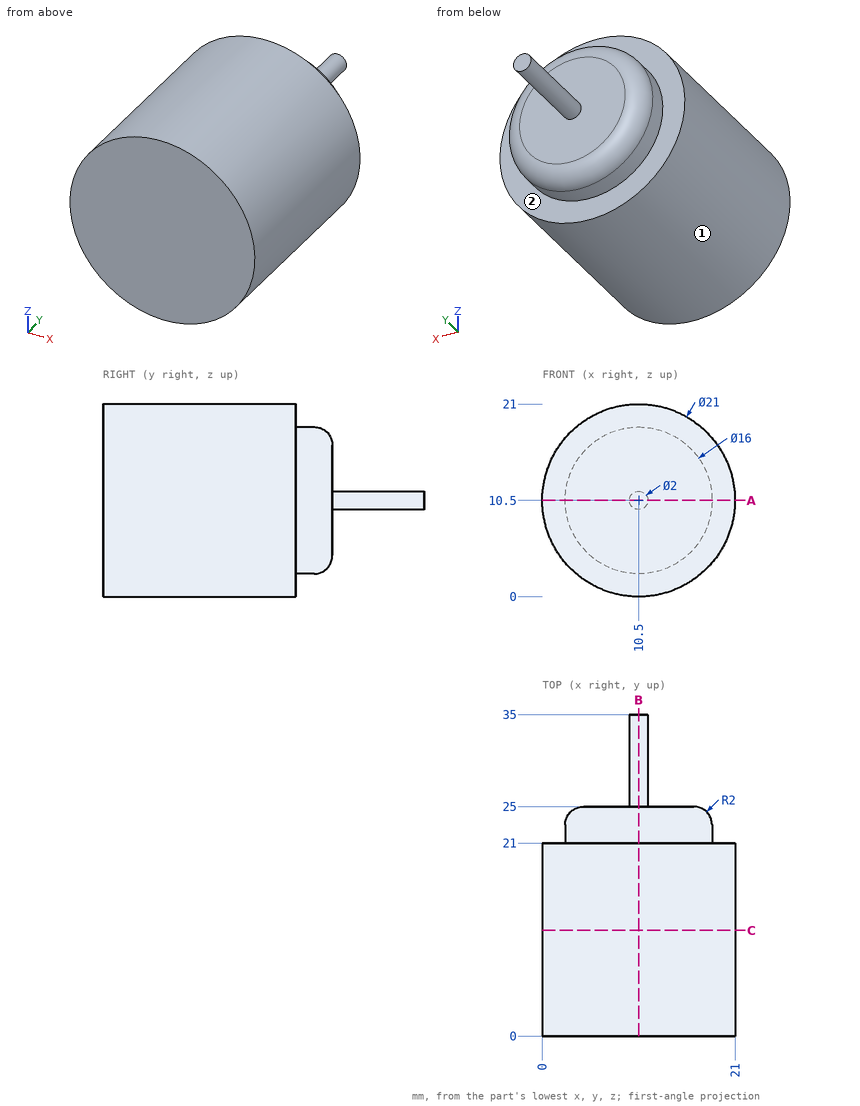
Study the drawing (mm; zero at the part's minimum x, y, z) and answer. A direction names the side the tool comes from. Coordinates: 2 decimals unless noted, no trailing zeros. Loops run counter-clockwise (first coordinate to the right, second up) from the corner with the lowest first, then second, coordinate; pieces in that order, holes last. Notation, with made-up numbers: (31, 1) -> (61, 1) arc R17 ccw to (61, 31) -> close; hole circle Ø6 at (73.5, 24). An arc over 180 degrees is marked (long way). Answer in a Markdown table with one row per item. Add a question column.
1. Consider line 1 (Y direction, x = 16.75, z = 3.5); line 2 (Y direction, x = 10, z = 4.75); line 3 (X direction, y = 33, z = 10.75). Determine where each line is inside the solid, lowest interval first. Write a range as [from, to].
2. The part is cut by section B-B, the plane x = 10.5. Write down the section's boundary in (y, z).
3. For the marked faces 1 and 2, determine the directions among +Z, -Z, +X, -X, +Y, -Y from which every point of the face is accessible in a straight line to the end or side of a thin tool.
4. The part is cut by section C-C, the plane y = 11.5. Write down the section's boundary in (x, z), then the cut area to 3 significant figures.
5. The part is cut by section A-A, the plane z = 10.5. Write down the section's boundary in (x, y).
6. Flat-ended cylindrical pins translate along their axes: P1, Ø4, axis at y = 8, z = 4.5, coming from the -X side; P2, Ø4, axis at y = 6, z = 13, coming from the -X side. Find the tip coordinate at first contact, or state that the pin passes through.
Answer below:
| question | item | result |
|---|---|---|
| 1 | line 1 | [0, 21] |
| 1 | line 2 | [0, 25] |
| 1 | line 3 | [9.53, 11.47] |
| 2 | outline | (0, 0) -> (21, 0) -> (21, 2.5) -> (23, 2.5) arc R2 ccw to (25, 4.5) -> (25, 9.5) -> (35, 9.5) -> (35, 11.5) -> (25, 11.5) -> (25, 16.5) arc R2 ccw to (23, 18.5) -> (21, 18.5) -> (21, 21) -> (0, 21) -> close |
| 3 | face 1 | +Y, -Y |
| 3 | face 2 | +Y |
| 4 | outline | circle Ø21 at (10.5, 10.5) |
| 4 | area | 346 mm2 |
| 5 | outline | (0, 0) -> (21, 0) -> (21, 21) -> (18.5, 21) -> (18.5, 23) arc R2 ccw to (16.5, 25) -> (11.5, 25) -> (11.5, 35) -> (9.5, 35) -> (9.5, 25) -> (4.5, 25) arc R2 ccw to (2.5, 23) -> (2.5, 21) -> (0, 21) -> close |
| 6 | P1 | x = 0.79 |
| 6 | P2 | x = 0.01 |
